Source: CAD feature listing. Evaluate the final solid. Frame: model axes, mm. A direction names the side the tool comes from. Give positions to 0.01 mm unless a question says otherwise; leave off trailing zeros. Write each loop counter-clockwise with the first axis right and the second up, starting at its lowest first coordinate (ties: lowest second). Pieces come first, ordered by that corner, then holes. Notation, with made-up numbers: M -33.75,-9.75 L -16.75,-9.75 A14 cw -16.75,-4.75 Z; hole C 73,26 d6. An arc over 180 degrees is marked long. Use CSV: the item, a comma, the result in double quotes. Start each with the question number.
from build123d import *

# Parameters (mm, degrees)
SKETCH_W     = 18
SKETCH_H     = 50
PAD_DEPTH    = 3
SKETCH002_R  = 2
POCKET_DEPTH = 5
PAD001_DEPTH = 25
CHAMFER_SIZE = 0.5


with BuildPart() as part:
    # Sketch → Pad (new body)
    with BuildSketch(Plane.XY):
        Rectangle(SKETCH_W, SKETCH_H)
    extrude(amount=PAD_DEPTH)

    # Sketch002 → Pocket (cut)
    with BuildSketch(Plane.XY.offset(3)):
        with Locations((0, 10)):
            Circle(SKETCH002_R)
        with Locations((0, -10)):
            Circle(SKETCH002_R)
        with Locations((0, 20)):
            Circle(SKETCH002_R)
        Circle(SKETCH002_R)
        with Locations((0, -20)):
            Circle(SKETCH002_R)
    extrude(amount=-POCKET_DEPTH, mode=Mode.SUBTRACT)

    # Sketch003 (on Face4 of Pocket) → Pad001 (join)
    with BuildSketch(Plane(origin=(0, 0, 0), x_dir=(1, 0, 0), z_dir=(0, 0, -1))):
        with BuildLine():
            ThreePointArc((9, -20), (14, 0), (9, 20))
            Line((9, 20), (9, -20))
        make_face()
    extrude(amount=-PAD001_DEPTH)

    # Chamfer
    chamfer_edges = [part.edges().sort_by_distance(p)[0] for p in [
        (0, 25, 0),
        (9, 22.5, 0),
        (14, 0, 0),
        (9, -22.5, 0),
        (0, -25, 0),
        (-9, 0, 0),
        (-2, -20, 0),
        (-2, 20, 0),
        (-2, -10, 0),
        (-2, 0, 0),
        (-2, 10, 0),
        (0, 25, 3),
        (-9, 0, 3),
        (0, -25, 3),
        (-2, 20, 3),
        (-2, 10, 3),
        (-2, 0, 3),
        (-2, -10, 3),
        (-2, -20, 3),
    ]]
    chamfer(chamfer_edges, length=CHAMFER_SIZE)


solid = part.part
1. Section C-C on z = 8.75. Return loops of the section in (x, y).
2. Pull-direction query (Y, two-part tool) for faces 4 (the flat face through (9, 22, 2)), 5 (the cylindrical face through (0, -18, 2)), 6 (the conical face through (13.634, 0.291, 0.135)); classes: released by +Y, released by -Y, zero draft, split by the parting line, or undercut.
3. Section A-A on y = 0. Return loops of the section in (x, z).
4. First-contact query: pin 1 (4 mm diameter, centred on x = 2, y = 19, fed in from -Z); pin 2 (6 mm diameter, centred on y = 9, z = 21, fed in from -X); pin 3 (4.5 mm diameter, centred on x = 0, y = -20, fed in from +Z); pin 4 (0.8 mm diameter, centred on y = -22.5, z = 2, fed in from +X). Flat tips, straight axial feed; report the tip coordinate or a pass-through.
5. Section D-D on x = 0. Give the number of separate pieces and of enclosed holes in the cut face, then the cut area to 3 significant figures.
6. Line query: probe 1 along Y at (x, z) = (0, 2.1); probe 2 along Z at (x, y) = (-5.5, -18.5); probe 3 along X at (y, z) = (7, 10.25). Output: solid intervals per line, ascending.
7. Access query for faces 1 (the cylindrical face through (0, -8, 2)), 2 (the flat face through (9, 0, 14)), 3 (the flat face through (9, -23, 2)). Directions: +Z, -Z, +X, -X, +Y, -Y. A direction counts if a zero-diameter tool reaches every point of the face in a straight line with its end or side. Return the directions, or none.
8. Section B-B on x = -4.5. Return loops of the section in (y, z).
Resolved:
1,outline,"M 9,-20 A42.5 ccw 9,20 Z"
2,face 4,"zero draft"
2,face 5,"undercut"
2,face 6,"split by the parting line"
3,outline,"M -9,0.5 L -8.5,0 L -2.5,0 L -2,0.5 L -2,2.5 L -2.5,3 L -8.5,3 L -9,2.5 Z; M 2,0.5 L 2.5,0 L 13.5,0 L 14,0.5 L 14,25 L 9,25 L 9,3 L 2.5,3 L 2,2.5 Z"
4,pin 1,"stops at z = 0"
4,pin 2,"stops at x = 9"
4,pin 3,"stops at z = 2.75"
4,pin 4,"stops at x = 9"
5,separate pieces,"6"
5,enclosed holes,"0"
5,area,"87.0 mm2"
6,probe 1,"y = -25 to -22, -18 to -12, -8 to -2, 2 to 8, 12 to 18, 22 to 25"
6,probe 2,"z = 0 to 3"
6,probe 3,"x = 9 to 13.42"
7,face 1,"+Z, -Z"
7,face 2,"+Z, -X, +Y, -Y"
7,face 3,"+Z, -Z, +X, -Y"
8,outline,"M -25,0.5 L -24.5,0 L 24.5,0 L 25,0.5 L 25,2.5 L 24.5,3 L -24.5,3 L -25,2.5 Z"
